Autodesk Inventor part; units mm, degrees
ref_plane "YZ Plane" through (0, 0, 0) normal (1, 0, 0) x (0, 1, 0)
ref_plane "XZ Plane" through (0, 0, 0) normal (0, 1, 0) x (-1, 0, 0)
ref_plane "XY Plane" through (0, 0, 0) normal (0, 0, 1) x (1, 0, 0)
sketch "Boceto3" plane through (0, 0, 0) normal (0, 0, 1) x (1, 0, 0)
  line L0 (0, 0) -> (180, 0)
  line L1 (180, 0) -> (180, 90)
  line L2 (180, 90) -> (0, 90)
  line L3 (0, 90) -> (0, 0)
  circle A0 centre (35, 50) radius 11
  circle A1 centre (70.8, 50) radius 11
  circle A2 centre (106.6, 50) radius 11
  circle A3 centre (142.4, 50) radius 11
  circle A4 centre (15, 10) radius 2.5
  dimension "d1" = 90
  dimension "d3" = 22
  dimension "d4" = 50
  dimension "d6" = 35.8
  dimension "d7" = 35.8
  dimension "d8" = 35.8
  dimension "d9" = 35
  dimension "d37" = 5
  dimension "d38" = 10
  dimension "d39" = 15
  dimension "d40" = 180
extrude "Extrusión1" add sketch "Boceto3" along normal blind 6
sketch "Boceto4" plane through (0, 0, 6) normal (0, 0, 1) x (1, 0, 0)
  line L0 (36, 12) -> (44, 12)
  line L1 (44, 12) -> (44, 8.9)
  line L2 (36, 8.9) -> (36, 12)
  line L3 (0, 0) -> (180, 0)
  line L4 (42.5, 8.9) -> (42.5, 0)
  line L5 (37.5, 0) -> (37.5, 8.9)
  line L6 (44, 8.9) -> (42.5, 8.9)
  line L7 (37.5, 8.9) -> (36, 8.9)
  line L8 (37.5, 0) -> (42.5, 0)
  line L9 (180, 90) -> (0, 90)
  line L10 (90, 90) -> (90, 0)
  line L11 (144, 12) -> (136, 12)
  line L12 (136, 12) -> (136, 8.9)
  line L13 (144, 8.9) -> (144, 12)
  line L14 (137.5, 8.9) -> (137.5, 0)
  line L15 (142.5, 0) -> (142.5, 8.9)
  line L16 (136, 8.9) -> (137.5, 8.9)
  line L17 (142.5, 8.9) -> (144, 8.9)
  line L18 (142.5, 0) -> (137.5, 0)
  point P0 (40, 12)
  point P1 (40, 0)
  point P2 (140, 12)
  point P3 (140, 0)
  point P4 (137.5, 0)
  point P5 (142.5, 0)
  dimension "d12" = 8
  dimension "d13" = 3.1
  dimension "d14" = 5
  dimension "d15" = 12
  dimension "d16" = 40
sketch "Boceto5" plane through (0, 0, 0) normal (0, -1, 0) x (1, 0, 0)
  line L0 (180, 6) -> (0, 6)
  line L1 (180, 0) -> (0, 0)
  line L2 (30, 6) -> (20, 6)
  line L3 (20, 6) -> (20, 0)
  line L4 (20, 0) -> (30, 0)
  line L5 (30, 0) -> (30, 6)
  line L6 (50, 6) -> (60, 6)
  line L7 (60, 6) -> (60, 0)
  line L8 (60, 0) -> (50, 0)
  line L9 (50, 0) -> (50, 6)
  line L10 (90, 6) -> (90, 0)
  line L11 (150, 6) -> (160, 6)
  line L12 (160, 6) -> (160, 0)
  line L13 (160, 0) -> (150, 0)
  line L14 (150, 0) -> (150, 6)
  line L15 (130, 6) -> (120, 6)
  line L16 (120, 6) -> (120, 0)
  line L17 (120, 0) -> (130, 0)
  line L18 (130, 0) -> (130, 6)
  point P0 (150, 6)
  point P1 (150, 0)
  point P2 (160, 0)
  point P3 (160, 6)
  point P4 (130, 0)
  point P5 (130, 6)
  point P6 (120, 6)
  point P7 (120, 0)
  point P8 (50, 0)
  point P9 (30, 0)
  point P10 (20, 6)
  dimension "d17" = 10
  dimension "d18" = 10
  dimension "d19" = 20
  dimension "d20" = 20
extrude "Extrusión2" cut sketch "Boceto4" against normal through all
extrude "Extrusión3" add sketch "Boceto5" along normal blind 3 contours L12 L1 L14 L0 | L18 L1 L16 L0 | L7 L1 L9 L0 | L5 L1 L3 L0
sketch "Boceto7" plane through (0, 0, 6) normal (0, 0, 1) x (1, 0, 0)
  line L0 (0, 78) -> (6, 78)
  line L1 (6, 78) -> (6, 63)
  line L2 (6, 63) -> (0, 63)
  line L3 (180, 90) -> (0, 90)
  line L4 (0, 90) -> (0, 0)
  line L5 (180, 0) -> (180, 90)
  line L6 (0, 45) -> (180, 45)
  line L7 (90, 90) -> (90, 0)
  line L8 (60, 0) -> (120, 0)
  line L9 (0, 12) -> (6, 12)
  line L10 (6, 12) -> (6, 27)
  line L11 (6, 27) -> (0, 27)
  line L12 (180, 78) -> (174, 78)
  line L13 (174, 78) -> (174, 63)
  line L14 (174, 63) -> (180, 63)
  line L15 (180, 12) -> (174, 12)
  line L16 (174, 12) -> (174, 27)
  line L17 (174, 27) -> (180, 27)
  point P0 (0, 27)
  point P1 (180, 12)
  point P2 (180, 27)
  point P3 (180, 63)
  point P4 (180, 78)
  dimension "d31" = 6
  dimension "d32" = 15
  dimension "d33" = 12
extrude "Extrusión5" cut sketch "Boceto7" against normal through all contours L5 L15 L16 L17 | L11 L10 L9 L4 | L0 L1 L2 L4 | L5 L14 L13 L12
properties part number "CaraLateral"
Input: part model. Units: mm. Frame: model coordinates. A direction names the side the tool comes from. Coordinates: 2 decimals unless noted, no trailing zeros. Write each loop counter-clockwise with the first axis right and the second up, starting at its lowest first coordinate (ties: lowest second). Pieces come first, ordered by that corner, then holes. Notation, with made-up numbers: (-31, 17.5) - (7, 17.5) arc R8 ccw to (7, 31.5) - close; hole circle Ø3 at (50, 41.25). An arc over 180 degrees is marked (long way). Put each result on its own line as item: value. Start each with the question number.
1) Reachability of faces 4 (the face through (180, 6, 3)), 5 (the face through (6, 19, 3)), 6 (the face through (137.5, 5, 3)), 7 (the face through (174, 19, 3)), 8 (the face through (36, 10, 3)) from +Z, -Z, +X, -X, +Y, -Y: full face, straight path, thin tool, end or side. Return the list, or none.
2) Cut plane D-D (z = 1.55). State how many separate pieces and enclosed holes the cut face has, plus the area to 3 significant figures.
3) Ray query, L1, parallel to Y at x = 15, z = 4.5; L2, parallel to Y at x = 70.8, z = 3.5; L3, parallel to X at y = 54, z = 4.85. Return the intervals inside material, ascending.
4) Mould query, pull axis Y, two halves, no side actions, for faces 1 (the face through (3, 78, 3)), 2 (the face through (146, 0, 3)), 3 (the face through (180, 84, 3)). Classes: pulls with the +Y half, pulls with the -Y half, needs draft (parallel to the pull), parting line crosses it, or undercut.
5) Cut plane A-A (x = 70.8). Return the cut outline in (y, z).
6) Cut plane B-B (y = 50). Return the cut outline in (x, z).
7) Contact query for flat-ended pins moving along their axis: pin 1 (2.5 mm diameter, centred on y = -2, z = 2.5, fed in from -X); pin 2 (3.5 mm diameter, centred on y = 11, z = 3.5, fed in from -X); pin 3 (3 mm diameter, centred on x = 84, z = 3, fed in from -Y); pin 4 (1 mm diameter, centred on y = 21, z = 3, fed in from +X). Output: stop coordinate, or through.
8) Cut plane C-C (x = 15). Return the cut outline in (y, z), plus the area to 3 significant figures.
Resolved:
1. face 4: +Z, -Z, +X, +Y, -Y
1. face 5: +Z, -Z, -X
1. face 6: +Z, -Z, -Y
1. face 7: +Z, -Z, +X
1. face 8: +Z, -Z
2. separate pieces: 1
2. enclosed holes: 5
2. area: 14,300 mm2
3. L1: y = 0 to 7.5, 12.5 to 90
3. L2: y = 0 to 39, 61 to 90
3. L3: x = 0 to 24.75, 45.25 to 60.55, 81.05 to 96.35, 116.85 to 132.15, 152.65 to 180
4. face 1: undercut
4. face 2: pulls with the -Y half
4. face 3: needs draft
5. outline: (0, 0) - (39, 0) - (39, 6) - (0, 6) - close; (61, 0) - (90, 0) - (90, 6) - (61, 6) - close
6. outline: (0, 0) - (24, 0) - (24, 6) - (0, 6) - close; (46, 0) - (59.8, 0) - (59.8, 6) - (46, 6) - close; (81.8, 0) - (95.6, 0) - (95.6, 6) - (81.8, 6) - close; (117.6, 0) - (131.4, 0) - (131.4, 6) - (117.6, 6) - close; (153.4, 0) - (180, 0) - (180, 6) - (153.4, 6) - close
7. pin 1: stops at x = 20
7. pin 2: stops at x = 0
7. pin 3: stops at y = 0
7. pin 4: stops at x = 174
8. outline: (0, 0) - (7.5, 0) - (7.5, 6) - (0, 6) - close; (12.5, 0) - (90, 0) - (90, 6) - (12.5, 6) - close
8. area: 510 mm2
